```python
from build123d import *

# Parameters (mm, degrees)
F0_R     = 2.1
F1_DEPTH = 4.83
F2_SIZE2 = 2.5
F2_SIZE  = 3.5
F3_R     = 2
F4_R     = 2


with BuildPart() as f1:
    # F0 (on Top) → F1 (new body)
    with BuildSketch(Plane.XY):
        Polygon((-12.5, -6), (9, -6), (12.5, -2.5), (12.5, 2.5), (9, 6), (-12.5, 6), (-18.5, 6), (-18.5, -6), align=None)
        with Locations((-14.5, 0)):
            Circle(F0_R, mode=Mode.SUBTRACT)
        with BuildLine():
            Line((5, -2.6), (-5, -2.6))
            ThreePointArc((-5, -2.6), (-7.6, 0), (-5, 2.6))
            Line((-5, 2.6), (5, 2.6))
            ThreePointArc((5, 2.6), (7.6, 0), (5, -2.6))
        make_face(mode=Mode.SUBTRACT)
    extrude(amount=F1_DEPTH)

    # F2
    f2_edges = [f1.edges().sort_by_distance(p)[0] for p in [
        (12.5, 0, 4.83),
    ]]
    f2_side = f1.faces().sort_by_distance((-4.75, -5.667585, 4.83))[0]
    chamfer(f2_edges, length=F2_SIZE, length2=F2_SIZE2, reference=f2_side)

    # F3
    f3_edges = [f1.edges().sort_by_distance(p)[0] for p in [
        (-18.5, -6, 2.415),
    ]]
    fillet(f3_edges, radius=F3_R)

    # F4
    f4_edges = [f1.edges().sort_by_distance(p)[0] for p in [
        (-18.5, 6, 2.415),
    ]]
    fillet(f4_edges, radius=F4_R)


solid = f1.part
```
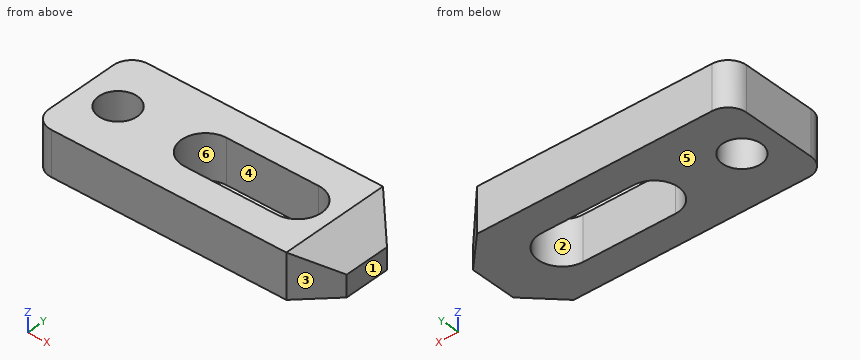
Source: CAD feature listing. Evaluate the final solid. Frame: model axes, mm. Face numbers are marked on the shaded views. A direction names the side the tool comes from. Round coordinates to 2 decimals unless told otherwise and drop trailing zeros. Loops run counter-clockwise (first coordinate to the right, second up) from the corner with the lowest first, then second, coordinate; pieces in that order, holes last. Notation, with made-up numbers: M 24,28 L 35,28 A14 ccw 35,53 Z; hole C -40,85 d4. An arc over 180 degrees is marked long. Use a Markdown table: item, result. Add a question column.
1. Section query C-C on y = 0. Return the cut outline in (x, z), then the cut area to 3 significant figures.
2. Section query B-B on x = 4. Return the cut outline in (y, z), then the cut area to 3 significant figures.
3. Mould query, pull axis Y, two halves, no side actions, for the marked faces 3, 4, 5 and 6. Classes: pulls with the +Y half, pulls with the -Y half, needs draft (parallel to the pull), parting line crosses it, or undercut.
4. Line query: line 1 (Y direction, x = -14.5, z = 1.95); line 2 (X direction, y = -1.75, z = 0.55); line 3 (Y direction, x = 4, z = 2.95). Output: solid intervals per line, ascending.
5. Section query D-D on x = -14.5. Return the cut outline in (y, z), then the cut area to 3 significant figures.
6. Section query A-A on z = 0.5. Return the cut outline in (x, y).
7. Contact query for a flat-ended pin moving along its axis: P1, Ø4, axis at x = -14.5, y = 0, coming from the -Z side. Output: stop coordinate, or through.
8. Reachability of the marked faces 1 and 2 from +Z, -Z, +X, -X, +Y, -Y: full face, straight path, thin tool, end or side. Return the list, or none.
Reported:
| question | item | result |
|---|---|---|
| 1 | outline | M -18.5,0 L -16.6,0 L -16.6,4.83 L -18.5,4.83 Z; M -12.4,0 L -7.6,0 L -7.6,4.83 L -12.4,4.83 Z; M 7.6,0 L 12.5,0 L 12.5,2.33 L 9,4.83 L 7.6,4.83 Z |
| 1 | area | 51.7 mm² |
| 2 | outline | M -6,0 L -2.6,0 L -2.6,4.83 L -6,4.83 Z; M 2.6,0 L 6,0 L 6,4.83 L 2.6,4.83 Z |
| 2 | area | 32.8 mm² |
| 3 | face 3 | pulls with the -Y half |
| 3 | face 4 | undercut |
| 3 | face 5 | needs draft |
| 3 | face 6 | undercut |
| 4 | line 1 | y = -6 to -2.1, 2.1 to 6 |
| 4 | line 2 | x = -18.5 to -15.66, -13.34 to -6.92, 6.92 to 12.5 |
| 4 | line 3 | y = -6 to -2.6, 2.6 to 6 |
| 5 | outline | M -6,0 L -2.1,0 L -2.1,4.83 L -6,4.83 Z; M 2.1,0 L 6,0 L 6,4.83 L 2.1,4.83 Z |
| 5 | area | 37.7 mm² |
| 6 | outline | M -18.5,-4 A2 ccw -16.5,-6 L 9,-6 L 12.5,-2.5 L 12.5,2.5 L 9,6 L -16.5,6 A2 ccw -18.5,4 Z; hole C -14.5,0 d4.2; hole M -5,-2.6 L 5,-2.6 A2.6 ccw 5,2.6 L -5,2.6 A2.6 ccw Z |
| 7 | P1 | passes through |
| 8 | face 1 | +Z, -Z, +X, +Y, -Y |
| 8 | face 2 | +Z, -Z |
